```python
from build123d import *

# Parameters (mm, degrees)
BOSS_EXTRUDE1_DEPTH = 2
SKETCH2_R           = 1.5
CUT_EXTRUDE1_DEPTH  = 2
SKETCH3_R           = 3
SKETCH3_R_2         = 4
CUT_EXTRUDE2_DEPTH  = 10
FILLET1_R           = 3


with BuildPart() as part:
    # Sketch1 → Boss-Extrude1 (new body)
    with BuildSketch(Plane.XY):
        with BuildLine():
            Line((35, 35), (35, 65))
            ThreePointArc((35, 65), (30, 70), (25, 65))
            Line((25, 65), (25, 35))
            Line((25, 35), (-35, 35))
            Line((-35, 35), (-35, -35))
            Line((-35, -35), (35, -35))
            Line((35, -35), (35, 35))
        make_face()
    extrude(amount=BOSS_EXTRUDE1_DEPTH)

    # Sketch2 → Cut-Extrude1 (cut)
    with BuildSketch(Plane.XY.offset(2)):
        with Locations((30, 65)):
            Circle(SKETCH2_R)
    extrude(amount=-CUT_EXTRUDE1_DEPTH, mode=Mode.SUBTRACT)

    # Sketch3 → Cut-Extrude2 (cut)
    with BuildSketch(Plane.XY.offset(2)):
        with Locations((0, 25)):
            Circle(SKETCH3_R)
        with Locations((25, 25)):
            Circle(SKETCH3_R)
        with Locations((25, 0)):
            Circle(SKETCH3_R)
        with Locations((25, -25)):
            Circle(SKETCH3_R)
        with Locations((0, -25)):
            Circle(SKETCH3_R)
        with Locations((-25, -25)):
            Circle(SKETCH3_R)
        with Locations((-25, 0)):
            Circle(SKETCH3_R)
        with Locations((-25, 25)):
            Circle(SKETCH3_R)
        with Locations((-20, -10)):
            Circle(SKETCH3_R_2)
        with Locations((20, 10)):
            Circle(SKETCH3_R_2)
    extrude(amount=-CUT_EXTRUDE2_DEPTH, mode=Mode.SUBTRACT)

    # Fillet1
    fillet1_edges = [part.edges().sort_by_distance(p)[0] for p in [
        (35, -35, 1),
        (-35, -35, 1),
        (-35, 35, 1),
        (25, 35, 1),
    ]]
    fillet(fillet1_edges, radius=FILLET1_R)


solid = part.part
```
Here's how the part is built. I have some questions about the finished solid (model axes, mm). A direction names the side the tool comes from. Coordinates: 2 decimals unless noted, no trailing zeros. Order: outer loops, then holes, each group sorted by start corner. A loop starts at its lowest first (then second) coordinate and runs counter-clockwise, first axis right, second up. Notation, with made-up numbers: (30, 81.25) - (57, 81.25) arc R11 cw to (57, 99.25) - close; hole circle Ø2 at (75.5, 79). An arc over 180 degrees is marked (long way). One line per question, with ' | ' between items.
(1) If I drill on L1, parallel to Y at x = 0, z = 1.35; L2, parallel to Y at x = -25, z = 1; L3, parallel to Y at x = 27.5, z = 0.1, over which ranges is the centre line in solid material (lowest first)?
Report:
L1: y = -35 to -28, -22 to 22, 28 to 35 | L2: y = -35 to -28, -22 to -3, 3 to 22, 28 to 35 | L3: y = -35 to -26.66, -23.34 to -1.66, 1.66 to 23.34, 26.66 to 69.33
(2) If we mould it in two halves opening along X, with no side actions, what happens to faces 1 (the flat face through (0, 7, 0)), 2 (the flat face through (-35, 0, 1)), 3 (the cylindrical face through (28.5, 65.07, 1.01))? For each: pulls with the +X half, pulls with the -X half, needs draft (parallel to the pull), parting line crosses it, or undercut.
Report:
face 1: needs draft | face 2: pulls with the -X half | face 3: undercut
(3) Suppose I cut it at D-D on x = 11.5. List the corners of the cut face in (y, z) for me.
Report:
outline: (-35, 0) - (35, 0) - (35, 2) - (-35, 2) - close
(4) Suppose I cut it at B-B on z = 0.55. State how many separate pieces and enclosed holes the cut face has, and give its area (3 significant figures).
Report:
separate pieces: 1 | enclosed holes: 11 | area: 4,900 mm2
(5) For faces 4 (the flat face through (0, -35, 1)), 5 (the flat face through (25, 52, 1)), which set-ups out of +Z, -Z, +X, -X, +Y, -Y let a thin tool reach every point of the face, with its end or its side?
Report:
face 4: +Z, -Z, +X, -X, -Y | face 5: +Z, -Z, -X, +Y
(6) Suppose I cut it at A-A on y = 0. List the corners of the cut face in (x, z) for me.
Report:
outline: (-35, 0) - (-28, 0) - (-28, 2) - (-35, 2) - close; (-22, 0) - (22, 0) - (22, 2) - (-22, 2) - close; (28, 0) - (35, 0) - (35, 2) - (28, 2) - close
(7) Suppose I cut it at C-C on y = -25. List the corners of the cut face in (x, z) for me, and give its area (3 significant figures).
Report:
outline: (-35, 0) - (-28, 0) - (-28, 2) - (-35, 2) - close; (-22, 0) - (-3, 0) - (-3, 2) - (-22, 2) - close; (3, 0) - (22, 0) - (22, 2) - (3, 2) - close; (28, 0) - (35, 0) - (35, 2) - (28, 2) - close | area: 104 mm2
(8) Will these pins go through, and if not, where does the flat tip stop? pin 1 (12 mm diameter, centred on x = 27.5, y = -22, fed in from -Z); pin 2 (0.6 mm diameter, centred on x = -3.5, z = 1, fed in from +Y); pin 3 (0.6 mm diameter, centred on y = 53, z = 1.5, fed in from -X).
Report:
pin 1: stops at z = 0 | pin 2: stops at y = 35 | pin 3: stops at x = 25
